The listing builds one solid part. Answer for the finished solid, in the listing's coordinates (mm). A direction names the side the tool comes from. Coordinates: 2 decimals unless noted, no trailing zeros. Loops run counter-clockwise (first coordinate to the right, second up) from the corner with the lowest first, then second, coordinate; pieces in that order, holes last. Notation, with made-up numbers: (58, 79) - (105, 79) arc R22 ccw to (105, 107) - close; hole circle Ø8 at (19, 19.5). An arc over 180 degrees is marked (long way). Use one line per item in the form item = value. Start each with the question number.
```python
from build123d import *

# Parameters (mm, degrees)
F1_DEPTH       = 6.35
F2_R           = 3.81
F3_DEPTH       = 6.35
F5_D           = 2.032
F5_CSINK_D     = 3.81
F5_CSINK_ANGLE = 100
F7_D           = 2.032


with BuildPart() as f1:
    # F0 (on Top) → F1 (new body)
    with BuildSketch(Plane.XY):
        with BuildLine():
            ThreePointArc((-5.08, -26.9184786366), (-3.5921024484, -30.5105810851), (0, -31.9984786366))
            Line((0, -31.9984786366), (0, -26.9184786366))
            Line((0, -26.9184786366), (0, -21.8384786366))
            ThreePointArc((0, -21.8384786366), (-3.5921024484, -23.3263761882), (-5.08, -26.9184786366))
        make_face()
        with BuildLine():
            Line((0, -26.9184786366), (0, -31.9984786366))
            ThreePointArc((0, -31.9984786366), (3.5921024484, -30.5105810851), (5.08, -26.9184786366))
            ThreePointArc((5.08, -26.9184786366), (3.5921024484, -23.3263761882), (0, -21.8384786366))
            Line((0, -21.8384786366), (0, -26.9184786366))
        make_face()
        with BuildLine():
            ThreePointArc((5.08, -26.9184786366), (3.5921024484, -30.5105810851), (0, -31.9984786366))
            ThreePointArc((0, -31.9984786366), (-3.5921024484, -30.5105810851), (-5.08, -26.9184786366))
            Line((-5.08, -26.9184786366), (-5.08, -39.6184786366))
            ThreePointArc((-5.08, -39.6184786366), (0, -44.6984786366), (5.08, -39.6184786366))
            Line((5.08, -39.6184786366), (5.08, -26.9184786366))
        make_face()
        with BuildLine():
            ThreePointArc((0, -21.8384786366), (3.5921024484, -23.3263761882), (5.08, -26.9184786366))
            Line((5.08, -26.9184786366), (5.08, -6.8815904984))
            Line((5.08, -6.8815904984), (4.2115108686, -8.1691785863))
            ThreePointArc((4.2115108686, -8.1691785863), (2.384915539, -9.8138524083), (0, -10.4084786366))
            Line((0, -10.4084786366), (0, -21.8384786366))
        make_face()
        with BuildLine():
            Line((-5.08, -5.3284786366), (-5.08, -26.9184786366))
            ThreePointArc((-5.08, -26.9184786366), (-3.5921024484, -23.3263761882), (0, -21.8384786366))
            Line((0, -21.8384786366), (0, -10.4084786366))
            ThreePointArc((0, -10.4084786366), (-3.5921024484, -8.9205810851), (-5.08, -5.3284786366))
        make_face()
        with BuildLine():
            Line((5.08, -5.3284786366), (5.08, -6.8815904984))
            Line((5.08, -6.8815904984), (26.9371104656, 25.5229083624))
            ThreePointArc((26.9371104656, 25.5229083624), (25.5662995467, 32.5751191806), (18.5140887285, 31.2043082616))
            Line((18.5140887285, 31.2043082616), (-4.2115108686, -2.487778687))
            ThreePointArc((-4.2115108686, -2.487778687), (-0.9693096965, -0.3418125447), (2.8406999496, -1.116967768))
            ThreePointArc((2.8406999496, -1.116967768), (4.4853737717, -2.9435630977), (5.08, -5.3284786366))
        make_face()
        with BuildLine():
            Line((4.2115108686, -8.1691785863), (5.08, -6.8815904984))
            Line((5.08, -6.8815904984), (5.08, -5.3284786366))
            ThreePointArc((5.08, -5.3284786366), (4.4853737717, -2.9435630977), (2.8406999496, -1.116967768))
            Line((2.8406999496, -1.116967768), (0, -5.3284786366))
            Line((0, -5.3284786366), (0, -10.4084786366))
            ThreePointArc((0, -10.4084786366), (2.384915539, -9.8138524083), (4.2115108686, -8.1691785863))
        make_face()
        with BuildLine():
            ThreePointArc((-4.2115108686, -2.487778687), (-4.8580281603, -3.8432303766), (-5.08, -5.3284786366))
            ThreePointArc((-5.08, -5.3284786366), (-3.5921024484, -8.9205810851), (0, -10.4084786366))
            Line((0, -10.4084786366), (0, -5.3284786366))
            Line((0, -5.3284786366), (2.8406999496, -1.116967768))
            ThreePointArc((2.8406999496, -1.116967768), (-0.9693096965, -0.3418125447), (-4.2115108686, -2.487778687))
        make_face()
    extrude(amount=F1_DEPTH)

    # F2 (on face) → F3 (join)
    with BuildSketch(Plane.XY.offset(6.35)):
        with Locations((0, -26.9184786366)):
            Circle(F2_R)
    extrude(amount=F3_DEPTH)

    # F5 (through all)
    with Locations(Plane.XY.offset(12.7)):
        with Locations((0, -26.9184786366)):
            CounterSinkHole(F5_D / 2, F5_CSINK_D / 2, counter_sink_angle=F5_CSINK_ANGLE)

    # F7 (through all)
    with Locations(Plane.XY.offset(6.35)):
        with Locations((0, -39.6184786366)):
            Hole(F7_D / 2)


solid = f1.part
```
(1) A cutting plane is placed at A-A (x = 0). Determine the outline of the cut face in (y, z).
(2) Find the intervals of material crossed by probe 1 along Y at (x, z) = (0, 1.5); probe 2 along Z at (x, y) = (5.5, 5); probe 3 along X at (y, z) = (-7, 6), in increasing order. Write a range as from..to.
(3) A cutting plane is placed at B-B (y = -37). Determine the outline of the cut face in (x, z).
(4) A cutting plane is placed at D-D (x = 16). Determine the outline of the cut face in (y, z).
(5) Determine the mould class of faces 4 (the face through (15.856, 9.094, 3.131)), 5 (the face through (7.6, -2.6, 0)), 6 (the face through (0.13, -38.61, 3.13)) for opening direction Y: +Y half, -Y half, draft (parallel to the pull), parting line (faces both ways), or undercut.
(6) Each of these flat-tipped pins is pushed along its axis until it touches: pin 1 Ø3.5 at (x, y) = (0, -39.62) entering from +Z; pin 2 Ø6 at (y, z) = (12.5, 3.5) entering from +X; pin 3 Ø3 at (y, z) = (0.5, 2) entering from -X. Where does it stop, or does it pass through?
(7) For faces 1 (the face through (-2, -28, 12.7)), 2 (the face through (5.08, -23, 3)), 3 (the face through (-0.826, -30.638, 9.481)), determine the directions among +Z, -Z, +X, -X, +Y, -Y from which every point of the face is accessible in a straight line to the end or side of a thin tool.
(8) A cutting plane is placed at C-C (z = 7.75). Determine the outline of the cut face in (x, y), then the cut area to 3 significant figures.
Evaluation:
q1.outline = (-44.7, 0) - (-40.63, 0) - (-40.63, 6.35) - (-44.7, 6.35) - close; (-38.6, 0) - (-27.93, 0) - (-27.93, 11.95) - (-28.82, 12.7) - (-30.73, 12.7) - (-30.73, 6.35) - (-38.6, 6.35) - close; (-25.9, 0) - (3.76, 0) - (3.76, 6.35) - (-23.11, 6.35) - (-23.11, 12.7) - (-25.01, 12.7) - (-25.9, 11.95) - close
q2.probe_1 = -44.7..-40.63, -38.6..-27.93, -25.9..3.76
q2.probe_2 = 0..6.35
q2.probe_3 = -5.08..5.08
q3.outline = (-5.08, 0) - (5.08, 0) - (5.08, 6.35) - (-5.08, 6.35) - close
q4.outline = (9.31, 0) - (27.48, 0) - (27.48, 6.35) - (9.31, 6.35) - close
q5.face_4 = -Y half
q5.face_5 = draft
q5.face_6 = undercut
q6.pin_1 = 6.35
q6.pin_2 = 20.18
q6.pin_3 = -3.21
q7.face_1 = +Z, +X, -X, +Y, -Y
q7.face_2 = +Z, -Z, +X, -Y
q7.face_3 = +Z
q8.outline = circle Ø7.62 at (0, -26.92); hole circle Ø2.03 at (0, -26.92)
q8.area = 42.4 mm^2
